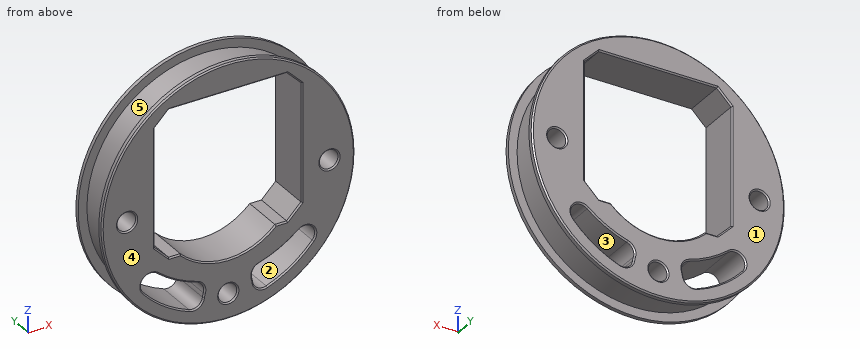
from build123d import *

# Parameters (mm, degrees)
SKETCH1_R               = 37.5
SKETCH1_R_2             = 2.75
BOSS_EXTRUDE1_DEPTH     = 6.5
SKETCH2_R               = 44.9
SKETCH2_R_2             = 34.9
CUT_EXTRUDE_THIN1_DEPTH = 5
CHAMFER1_SIZE           = 0.4
CHAMFER2_SIZE           = 0.4


with BuildPart() as part:
    # Sketch1 → Boss-Extrude1 (new body, symmetric)
    with BuildSketch(Plane(origin=(0, 0, 0), x_dir=(1, 0, 0), z_dir=(0, 1, 0))):
        Circle(SKETCH1_R)
        with Locations((0, 30)):
            Circle(SKETCH1_R_2, mode=Mode.SUBTRACT)
        with Locations((30, 0)):
            Circle(SKETCH1_R_2, mode=Mode.SUBTRACT)
        with Locations((-30, 0)):
            Circle(SKETCH1_R_2, mode=Mode.SUBTRACT)
        with BuildLine():
            Line((-17.494426356, 14.25), (-14.033442201, 14.25))
            ThreePointArc((-14.033442201, 14.25), (0, 20), (14.033442201, 14.25))
            Line((14.033442201, 14.25), (17.494426356, 14.25))
            Line((17.494426356, 14.25), (21.75, 9.994426356))
            Line((21.75, 9.994426356), (21.75, -24.994426356))
            Line((21.75, -24.994426356), (17.494426356, -29.25))
            Line((17.494426356, -29.25), (-17.494426356, -29.25))
            Line((-17.494426356, -29.25), (-21.75, -24.994426356))
            Line((-21.75, -24.994426356), (-21.75, 9.994426356))
            Line((-21.75, 9.994426356), (-17.494426356, 14.25))
        make_face(mode=Mode.SUBTRACT)
        with BuildLine():
            ThreePointArc((7.182286097, 27.840192967), (7.335670337, 28.438609369), (7.439285619, 29.047619048))
            ThreePointArc((7.439285619, 29.047619048), (8.853359783, 31.228166276), (11.439426083, 31.486338798))
            ThreePointArc((11.439426083, 31.486338798), (18.843045333, 27.698188435), (25.085377879, 22.203013684))
            ThreePointArc((25.085377879, 22.203013684), (24.997326571, 18.131103641), (20.931054397, 17.899511222))
            ThreePointArc((20.931054397, 17.899511222), (15.388292289, 21.593722157), (9.215229657, 24.09626166))
            ThreePointArc((9.215229657, 24.09626166), (7.418794885, 25.54470973), (7.182286097, 27.840192967))
        make_face(mode=Mode.SUBTRACT)
        with BuildLine():
            ThreePointArc((-25.085377879, 22.203013684), (-24.997326571, 18.131103641), (-20.931054397, 17.899511222))
            ThreePointArc((-20.931054397, 17.899511222), (-15.388292289, 21.593722157), (-9.215229657, 24.09626166))
            ThreePointArc((-9.215229657, 24.09626166), (-7.418794885, 25.54470973), (-7.182286097, 27.840192967))
            ThreePointArc((-7.182286097, 27.840192967), (-7.335670337, 28.438609369), (-7.439285619, 29.047619048))
            ThreePointArc((-7.439285619, 29.047619048), (-8.853359783, 31.228166276), (-11.439426083, 31.486338798))
            ThreePointArc((-11.439426083, 31.486338798), (-18.843045333, 27.698188435), (-25.085377879, 22.203013684))
        make_face(mode=Mode.SUBTRACT)
    extrude(amount=BOSS_EXTRUDE1_DEPTH, both=True)

    # Sketch2 → Cut-Extrude-Thin1 (cut, symmetric)
    with BuildSketch(Plane(origin=(0, 0, 0), x_dir=(1, 0, 0), z_dir=(0, 1, 0))):
        Circle(SKETCH2_R)
        Circle(SKETCH2_R_2, mode=Mode.SUBTRACT)
    extrude(amount=CUT_EXTRUDE_THIN1_DEPTH, both=True, mode=Mode.SUBTRACT)

    # Chamfer1
    chamfer1_edges = [part.edges().sort_by_distance(p)[0] for p in [
        (-37.5, -6.5, 0),
        (-37.5, 6.5, 0),
    ]]
    chamfer(chamfer1_edges, length=CHAMFER1_SIZE)

    # Chamfer2
    chamfer2_edges = [part.edges().sort_by_distance(p)[0] for p in [
        (-19.622213178, -6.5, -12.122213178),
        (-21.75, -6.5, 7.5),
        (-19.622213178, -6.5, 27.122213178),
        (0, -6.5, 29.25),
        (19.622213178, -6.5, 27.122213178),
        (21.75, -6.5, 7.5),
        (19.622213178, -6.5, -12.122213178),
        (15.763934278, -6.5, -14.25),
        (0, -6.5, -20),
        (-15.763934278, -6.5, -14.25),
        (-19.622213178, 6.5, -12.122213178),
        (-21.75, 6.5, 7.5),
        (-19.622213178, 6.5, 27.122213178),
        (0, 6.5, 29.25),
        (19.622213178, 6.5, 27.122213178),
        (21.75, 6.5, 7.5),
        (19.622213178, 6.5, -12.122213178),
        (15.763934278, 6.5, -14.25),
        (0, 6.5, -20),
        (-15.763934278, 6.5, -14.25),
        (-2.75, -6.5, -30),
        (-2.75, 6.5, -30),
        (27.25, -6.5, 0),
        (27.25, 6.5, 0),
        (-32.75, -6.5, 0),
        (-32.75, 6.5, 0),
        (-15.388292289, -6.5, -21.593722157),
        (-7.418794885, -6.5, -25.54470973),
        (-7.335670337, -6.5, -28.438609369),
        (-8.853359783, -6.5, -31.228166276),
        (-18.843045333, -6.5, -27.698188435),
        (-24.997326571, -6.5, -18.131103641),
        (-15.388292289, 6.5, -21.593722157),
        (-7.418794885, 6.5, -25.54470973),
        (-7.335670337, 6.5, -28.438609369),
        (-8.853359783, 6.5, -31.228166276),
        (-18.843045333, 6.5, -27.698188435),
        (-24.997326571, 6.5, -18.131103641),
        (18.843045333, -6.5, -27.698188435),
        (8.853359783, -6.5, -31.228166276),
        (7.335670337, -6.5, -28.438609369),
        (7.418794885, -6.5, -25.54470973),
        (15.388292289, -6.5, -21.593722157),
        (24.997326571, -6.5, -18.131103641),
        (18.843045333, 6.5, -27.698188435),
        (8.853359783, 6.5, -31.228166276),
        (7.335670337, 6.5, -28.438609369),
        (7.418794885, 6.5, -25.54470973),
        (15.388292289, 6.5, -21.593722157),
        (24.997326571, 6.5, -18.131103641),
    ]]
    chamfer(chamfer2_edges, length=CHAMFER2_SIZE)


solid = part.part
Here's how the part is built. I have some questions about the finished solid (model axes, mm). Face numbers are marked on the shaded views. A direction names the side the tool comes from. Coordinates: 2 decimals unless noted, no trailing zeros. Write each loop counter-clockwise with the first axis right and the second up, starting at its lowest first coordinate (ties: lowest second). Pieces come first, ordered by that corner, then holes.
Item 1: If I drill on line 1 (X direction, y = -3, z = 0); line 2 (Y direction, x = -28.5, z = 22); line 3 (X direction, y = -1.25, z = -30), over which ranges is the centre line in solid material (lowest first)?
Item 2: Will these pins go through, and if not, where does the flat tip stop? pin 1 (3.5 mm diameter, centred on y = 2.5, z = 11, fed in from +X); pin 2 (3 mm diameter, centred on x = -15, y = -3, fed in from +Z); pin 3 (1.5 mm diameter, centred on y = 1.5, z = 15.5, fed in from +X).
Item 3: I want a section at B-B on x = 0. Count the separate pieces of the cut face and the enclosed holes in it, and give its area (3 significant figures).
Item 4: I want a section at A-A on y = 1. Write out the boundary of the cut face in (x, z) (3 decimals).
Item 5: On a 3-axis mill with a long thin cutter (end or side, diameter ignored), from which of +Z, -Z, +X, -X, +Y, -Y can I reach the whole of each face in a straight line? I mean the marked faces 1 and 2. Say none if no direction works.
Item 6: If we mould it in two halves opening along X, with no side actions, what happens to the marked faces 3, 4 and 5? For each: +X half, -X half, draft (parallel to the pull), parting line (faces both ways), or undercut.
Findings below:
1. line 1: x = -34.9 to -32.75, -27.25 to -21.75, 21.75 to 27.25, 32.75 to 34.9
1. line 2: y = -6.5 to -5, 5 to 6.5
1. line 3: x = -17.83 to -14.91, -7.73 to -2.75, 2.75 to 7.73, 14.91 to 17.83
2. pin 1: stops at x = 33.65
2. pin 2: stops at z = 32.18
2. pin 3: stops at x = 31.63
3. separate pieces: 3
3. enclosed holes: 0
3. area: 210 mm2
4. outline: circle Ø69.8 at (0, 0); hole circle Ø5.5 at (-30, 0); hole (-25.085, -22.203) arc R33.5 ccw to (-11.439, -31.486) arc R3 ccw to (-7.439, -29.048) arc R7.5 cw to (-7.182, -27.84) arc R3 ccw to (-9.215, -24.096) arc R32.913 cw to (-20.931, -17.9) arc R3 ccw to start; hole (-21.75, -9.994) - (-17.494, -14.25) - (-14.033, -14.25) arc R20 ccw to (14.033, -14.25) - (17.494, -14.25) - (21.75, -9.994) - (21.75, 24.994) - (17.494, 29.25) - (-17.494, 29.25) - (-21.75, 24.994) - close; hole circle Ø5.5 at (0, -30); hole (7.182, -27.84) arc R7.5 cw to (7.439, -29.048) arc R3 ccw to (11.439, -31.486) arc R33.5 ccw to (25.085, -22.203) arc R3 ccw to (20.931, -17.9) arc R32.913 cw to (9.215, -24.096) arc R3 ccw to start; hole circle Ø5.5 at (30, 0)
5. face 1: +Z, -Z, +X, -X, +Y
5. face 2: +Y, -Y
6. face 3: undercut
6. face 4: draft
6. face 5: parting line
